Here's the drawing with two shaded views (mm, measured from the low corner). I have some questions. A direction names the side the tool comes from. Coordinates: 2 decimals unless noted, no trailing zeros. Loops run counter-clockwise (first coordinate to the right, second up) from the corner with the lowest first, then second, coordinate; pieces in that order, holes last. Notation, with made-up numbers: (58, -16) - (74, -16) arc R17 cw to (74, 1) - close; hole circle Ø9 at (79, 62.25). An arc over 180 degrees is marked (long way). One line per item, written item: value. Start each with the question number.
(1) If we section it at B-B on y = 19.5: Write out the boundary of the cut face in (x, z).
(2) If I drill on line 1 along Y through (x, z) = (2.6, 5.65); line 2 along Y through (x, z) = (10, 50.4); line 3 along Z through (x, y) = (3.75, 20), over which ranges is the centre line in solid material (lowest first)? Write a range as from..to.
(3) If we section it at C-C on x = 4: Write out the boundary of the cut face in (y, z).
(4) I'm going to push flat-ended pins straight in: P1, Ø5, axis at y = 50.5, z = 5.65, coming from the +X side; P2, Ø4, axis at x = 3, z = 19.5, coming from the -Y side; P3, Ø2.5, axis at x = 1.5, z = 32.5, coming from the +Y side. Where does each tip first touch, or does it pass through?
(5) On a 3-axis mill with a long thin cutter (end or side, diameter ignored), from which of +Z, -Z, +X, -X, +Y, -Y can I reach the whole of each face in a straight line? I mean the marked faces 5, 6 and 7. Say none if no direction works.
(6) If we mould it in two halves opening along Z, with no side actions, what happens to the marked faces 1, 2, 3 and 4? For each: pulls with the +Z half, pulls with the -Z half, needs draft (parallel to the pull), parting line crosses it, or undercut.
(7) If we section it at D-D on z = 5.65: Write out the boundary of the cut face in (x, y).
(8) If we section it at A-A on x = 10: Write out the boundary of the cut face in (y, z), then the cut area to 3 significant figures.
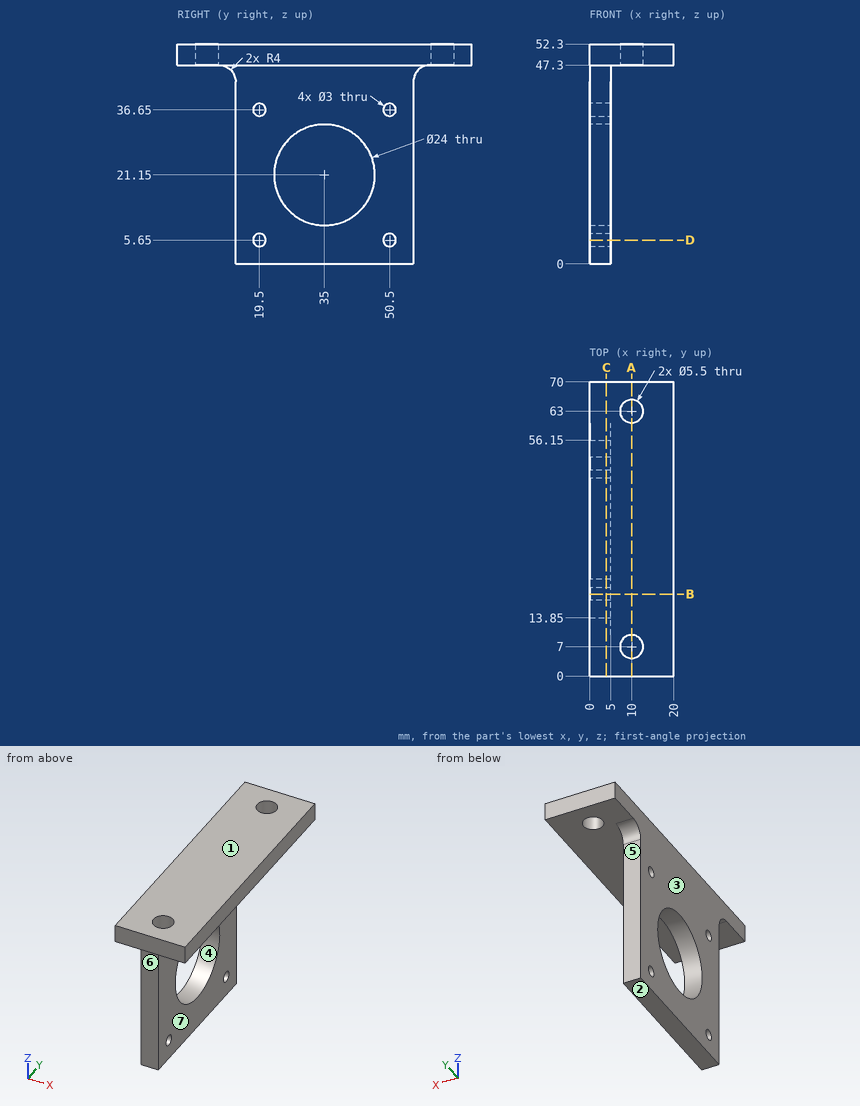
Values:
1. outline: (0, 0) - (5, 0) - (5, 4.15) - (0, 4.15) - close; (0, 7.15) - (5, 7.15) - (5, 35.15) - (0, 35.15) - close; (0, 38.15) - (5, 38.15) - (5, 47.3) - (20, 47.3) - (20, 52.3) - (0, 52.3) - close
2. line 1: y = 13.85..18, 21..49, 52..56.15
2. line 2: y = 0..4.25, 9.75..60.25, 65.75..70
2. line 3: z = 0..4.24, 7.06..35.24, 38.06..52.3
3. outline: (0, 47.3) - (9.85, 47.3) arc R4 cw to (13.85, 43.3) - (13.85, 0) - (56.15, 0) - (56.15, 43.3) arc R4 cw to (60.15, 47.3) - (70, 47.3) - (70, 52.3) - (0, 52.3) - close; hole circle Ø3 at (19.5, 5.65); hole circle Ø3 at (19.5, 36.65); hole circle Ø24 at (35, 21.15); hole circle Ø3 at (50.5, 5.65); hole circle Ø3 at (50.5, 36.65)
4. P1: stops at x = 5
4. P2: stops at y = 13.85
4. P3: stops at y = 56.15
5. face 5: -Z, +X, -X, +Y
5. face 6: -Z, +X, -X, -Y
5. face 7: -Z, +X, +Y, -Y
6. face 1: pulls with the +Z half
6. face 2: pulls with the -Z half
6. face 3: needs draft
6. face 4: undercut
7. outline: (0, 13.85) - (5, 13.85) - (5, 18) - (0, 18) - close; (0, 21) - (5, 21) - (5, 49) - (0, 49) - close; (0, 52) - (5, 52) - (5, 56.15) - (0, 56.15) - close
8. outline: (0, 47.3) - (4.25, 47.3) - (4.25, 52.3) - (0, 52.3) - close; (9.75, 47.3) - (60.25, 47.3) - (60.25, 52.3) - (9.75, 52.3) - close; (65.75, 47.3) - (70, 47.3) - (70, 52.3) - (65.75, 52.3) - close
8. area: 295 mm2
